Build history of the part. All positions in model axes, mm. A direction names the side the tool comes from. Coordinates: 2 decimals unless noted, no trailing zeros. Loops run counter-clockwise (first coordinate to the right, second up) from the corner with the lowest first, then second, coordinate; pieces in that order, holes last.
Item 1: Mould opens along X. For faces 4 (the face through (-5, 2, 0)), 5 (the face through (3, 4.5, 0)), 6 (the face through (5, 2, 0)), 7 (the face through (0.014, 3.375, 0.026)) say: released by +X, released by -X, zero draft, split by the parting line, or undercut.
Item 2: Cut at D-D (z = 2.25). List the corners of the cut face in (x, y).
Item 3: Cut at B-B (x = 1). List the corners of the cut face in (y, z).
Item 4: Cut at A-A (z = -1). List the corners of the cut face in (x, y) (3 decimals).
Item 5: Flat gauge pins, fed straight in: pin 1 (0.8 mm diameter, centred on x = 1.5, y = 4, fed in from -Z); pin 2 (1.1 mm diameter, centred on x = 1, z = -3.5, fed in from +Y). Where does each tip first touch, or does it go through?
Item 6: Cut at C-C (y = 2.85). List the corners of the cut face in (x, z).
Item 7: 3-axis set-ups, long thin cutter, end or side, ignore diameter. For faces 1 (the face through (0, 2, 3)), 2 (the face through (0, 2, -3)), 3 (the face through (0, 1, -4)): which of +Z, -Z, +X, -X, +Y, -Y reach the whole face in a straight line?
Item 8: Drill centre lines: line 1 along Y through (x, z) = (3, 2); line 2 along Z through (x, y) = (3.5, 3.4); line 3 along Y through (x, z) = (-0.25, -1). Where is each one in solid material? Low to high.
from build123d import *

# Parameters (mm, degrees)
SKETCH1_W           = 10
SKETCH1_H           = 8
BOSS_EXTRUDE1_DEPTH = 2
SKETCH2_W           = 10
SKETCH2_H           = 3.7
BOSS_EXTRUDE2_DEPTH = 2.5
CUT_EXTRUDE1_REACH  = 10.915


with BuildPart() as part:
    # Sketch1 → Boss-Extrude1 (new body)
    with BuildSketch(Plane(origin=(0, 0, 0), x_dir=(1, 0, 0), z_dir=(0, 1, 0))):
        Rectangle(SKETCH1_W, SKETCH1_H)
    extrude(amount=BOSS_EXTRUDE1_DEPTH)

    # Sketch2 → Boss-Extrude2 (add)
    with BuildSketch(Plane(origin=(0, 2, 0), x_dir=(1, 0, 0), z_dir=(0, 1, 0))):
        Rectangle(SKETCH2_W, SKETCH2_H)
    extrude(amount=BOSS_EXTRUDE2_DEPTH)

    # Sketch3 → Cut-Extrude1 (cut, up to next)
    with BuildSketch(Plane.XY.offset(1.85), mode=Mode.PRIVATE) as cut_extrude1_sk1:
        with BuildLine():
            Line((-0.625, 4), (-0.625, 4.5))
            Line((-0.625, 4.5), (0.625, 4.5))
            Line((0.625, 4.5), (0.625, 4))
            ThreePointArc((0.625, 4), (0, 3.375), (-0.625, 4))
        make_face()
    cut_extrude1_tool1 = extrude(cut_extrude1_sk1.sketch, amount=-CUT_EXTRUDE1_REACH, mode=Mode.PRIVATE) & part.part
    add(cut_extrude1_tool1.solids().sort_by_distance((0, 3.994744, 1.85))[0], mode=Mode.SUBTRACT)


solid = part.part
Filled sheet:
1. face 4: released by -X
1. face 5: zero draft
1. face 6: released by +X
1. face 7: undercut
2. outline: (-5, 0) - (5, 0) - (5, 2) - (-5, 2) - close
3. outline: (0, -4) - (2, -4) - (2, -1.85) - (4.5, -1.85) - (4.5, 1.85) - (2, 1.85) - (2, 4) - (0, 4) - close
4. outline: (-5, 0) - (5, 0) - (5, 4.5) - (0.625, 4.5) - (0.625, 4) arc R0.625 cw to (-0.625, 4) - (-0.625, 4.5) - (-5, 4.5) - close
5. pin 1: stops at z = -1.85
5. pin 2: stops at y = 2
6. outline: (-5, -1.85) - (5, -1.85) - (5, 1.85) - (-5, 1.85) - close
7. face 1: +Z, +X, -X, +Y
7. face 2: -Z, +X, -X, +Y
7. face 3: -Z, +X, -X, +Y, -Y
8. line 1: y = 0 to 2
8. line 2: z = -1.85 to 1.85
8. line 3: y = 0 to 3.43
